Design review of the part built by this model. Coordinates are the model's own, in mm. Face numbers are marked on the shaded views. Give positions to 0.01 mm unless a question says otherwise; leave off trailing zeros. Loops run counter-clockwise (first coordinate to the right, second up) from the corner with the lowest first, then second, coordinate; pieces in that order, holes last. Notation, with made-up numbers: (-31.75, 83.5) -> (10.25, 83.5) arc R34 ccw to (10.25, 121.5) -> close; hole circle Ø10 at (50.25, -38.5). An arc over 180 degrees is marked (long way). Answer in a Markdown table with one row per item. Add a question column.
(1) Consider section B-B on y = 19.2. Write out the cut boundary in (x, z).
(2) Draft analysis for pull direction X (two halves, no side actions). For the marked faces 1, 2 and 3, state which applies: +X half, -X half, draft (parallel to the pull), parting line (faces both ways), or undercut.
(3) For pin 1 (8 mm diameter, centred on y = 9, z = -1, fed in from -X); pin 2 (1 mm diameter, centred on y = 8, z = 9.5, fed in from +X); pin 3 (6 mm diameter, centred on x = 4, y = 7.5, fed in from +Z); pin 4 (2.5 mm diameter, centred on x = 0, y = 19.2, fed in from -Z), all flat-tipped, find the tip position at first contact; note any pin that passes through.
(4) For line 1 (Y direction, x = 0, z = 8.5); line 2 (Z direction, x = 0, y = 2); line 3 (Z direction, x = 3.75, y = 5), list the stretches that pass through material, from the lowest coordinate up.
(5) Consider section C-C on y = 22.75. Write out the cut boundary in (x, z), then the cut area to 3 significant figures.
(6) Consider section D-D on x = 6.5. Write out the cut boundary in (y, z), then the cut area to 3 significant figures.
(7) Consider section A-A on z = 0. Write out the cut boundary in (x, y), then the cut area to 3 significant figures.
Autodesk Inventor part; units mm, degrees
ref_plane "YZ Plane" through (0, 0, 0) normal (1, 0, 0) x (0, 1, 0)
ref_plane "XZ Plane" through (0, 0, 0) normal (0, 1, 0) x (-1, 0, 0)
ref_plane "XY Plane" through (0, 0, 0) normal (0, 0, 1) x (1, 0, 0)
sketch "Boceto1" plane through (0, 0, 0) normal (0, 1, 0) x (-1, 0, 0)
  circle A0 centre (0, 0) radius 12
  dimension "d0" = 24
extrude "Extrusión1" add sketch "Boceto1" along normal blind 25.6
sketch "Boceto2" plane through (0, 25.6, 0) normal (0, 1, 0) x (1, 0, 0)
  point P0 (0, 0)
  point P1 (0, 0)
hole "Agujero1" at (0, 25.6, 0) direction (0, -1, 0) diameter 5 depth 35 tip angle 118
sketch "Boceto3" plane through (0, 25.6, 0) normal (0, 1, 0) x (1, 0, 0)
  point P0 (0, 0)
  point P1 (0, 0)
hole "Agujero2" at (0, 25.6, 0) direction (0, -1, 0) diameter 8 depth 12.8
sketch "Boceto4" plane through (0, 0, 0) normal (1, 0, 0) x (0, 1, 0)
  line L0 (9.2, -7) -> (3.6, -7)
  line L1 (3.6, -7) -> (3.6, -9.42)
  line L2 (3.6, -9.42) -> (9.2, -9.42)
  line L3 (9.2, -9.42) -> (9.2, -7)
  line L4 (25.6, -12) -> (25.6, 12) construction
  line L5 (0, 12) -> (0, -12) construction
  line L6 (12.8, -2.5) -> (12.8, 2.5) construction
  line L7 (0, -2.5) -> (0, 2.5) construction
  line L8 (19.2, 26.4321) -> (19.2, -18.0419) construction
  line L9 (6.4, 12.9466) -> (6.4, -18.0419) construction
  line L10 (22, -7) -> (16.4, -7)
  line L11 (16.4, -7) -> (16.4, -9.42)
  line L12 (16.4, -9.42) -> (22, -9.42)
  line L13 (22, -9.42) -> (22, -7)
  line L14 (0, -2.5) -> (0, 2.5) construction
  point P0 (0, 0)
  point P1 (6.4, -7)
  point P2 (19.2, -7)
  dimension "d17" = 5.6
  dimension "d18" = 2.42
  dimension "d19" = 6.4
  dimension "d20" = 6.4
  dimension "d21" = 5.6
  dimension "d22" = 2.42
  dimension "d23" = 9.42
  dimension "d24" = 9.42
extrude "Extrusión2" cut sketch "Boceto4" along normal blind 10 and the other way blind 3
sketch "Boceto5" plane through (9.7468, 16.4, -7) normal (0, 0, -1) x (-1, 0, 0)
  line L0 (0, -7.2) -> (2.3128, -7.2) construction
  line L1 (2.3128, -7.2) -> (2.3128, -12.8) construction
  line L2 (2.3128, -12.8) -> (0, -12.8) construction
  line L3 (0, -12.8) -> (0, -7.2) construction
  line L4 (0, 5.6) -> (2.3128, 5.6) construction
  line L5 (2.3128, 5.6) -> (2.3128, 0) construction
  line L6 (2.3128, 0) -> (0, 0) construction
  line L7 (0, 0) -> (0, 5.6) construction
  line L8 (21.7468, 9.2) -> (-2.2532, 9.2) construction
  line L9 (-2.2532, -16.4) -> (21.7468, -16.4) construction
  point P0 (9.7468, -16.4)
  point P1 (9.7468, 2.8)
  point P2 (9.7468, -10)
  point P3 (2.3128, -10)
  point P4 (2.3128, 2.8)
hole "Agujero3" at (0, 19.2, -7) at (0, 6.4, -7) direction (0, 0, 1) diameter 3 end through all both
sketch "Boceto6" plane through (0, 12.8, 0) normal (0, 1, 0) x (1, 0, 0)
  circle A0 centre (0, 0) radius 4 construction
  circle A1 centre (0, 0) radius 12 construction
  circle A2 centre (0, 0) radius 2.5 construction
  line L0 (1.5, -1.5) -> (-1.5, -1.5)
  line L1 (-1.5, -1.5) -> (-1.5, 1.5)
  line L2 (-1.5, 1.5) -> (1.5, 1.5)
  line L3 (1.5, 1.5) -> (1.5, -1.5)
  line L4 (-1.5, 1.5) -> (1.5, -1.5) construction
  line L5 (1.5, 1.5) -> (-1.5, -1.5) construction
  circle A3 centre (0, 0) radius 4
  dimension "d36" = 3
  dimension "d37" = 3
  dimension "d38" = 8
extrude "Extrusión3" add sketch "Boceto6" along normal up to surface (12.8 mm away)
equation "\"d20\" = d19"
properties part number "Coupler 5x8"
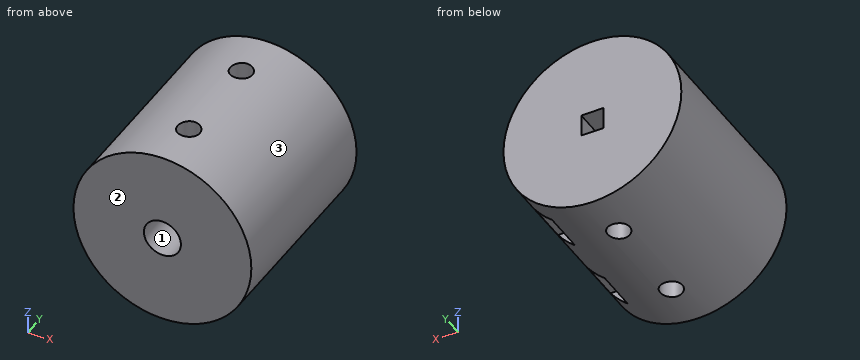
Values follow:
| question | item | result |
|---|---|---|
| 1 | outline | (-3, -9.42) -> (-3, -7) -> (-1.5, -7) -> (-1.5, -3.71) arc R4 ccw to (1.5, -3.71) -> (1.5, -7) -> (9.75, -7) arc R12 ccw to (1.5, 11.91) -> (1.5, 3.71) arc R4 ccw to (-1.5, 3.71) -> (-1.5, 11.91) arc R12 ccw to (-1.5, -11.91) -> (-1.5, -9.42) -> close; (1.5, -11.91) arc R12 ccw to (7.43, -9.42) -> (1.5, -9.42) -> close; hole (-1.5, -1.5) -> (1.5, -1.5) -> (1.5, 1.5) -> (-1.5, 1.5) -> close |
| 2 | face 1 | undercut |
| 2 | face 2 | draft |
| 2 | face 3 | parting line |
| 3 | pin 1 | x = -12 |
| 3 | pin 2 | x = 7.94 |
| 3 | pin 3 | z = 11.96 |
| 3 | pin 4 | z = -4 |
| 4 | line 1 | 0 to 4.9, 7.9 to 17.7, 20.7 to 25.6 |
| 4 | line 2 | -12 to -2.5, 2.5 to 12 |
| 4 | line 3 | -11.4 to -9.42, -7 to 11.4 |
| 5 | outline | circle Ø24 at (0, 0); hole (-1.5, -1.5) -> (1.5, -1.5) -> (1.5, 1.5) -> (-1.5, 1.5) -> close |
| 5 | area | 443 mm2 |
| 6 | outline | (0, -10.09) -> (25.6, -10.09) -> (25.6, 10.09) -> (0, 10.09) -> close; hole (3.6, -9.42) -> (9.2, -9.42) -> (9.2, -7) -> (3.6, -7) -> close; hole (16.4, -9.42) -> (22, -9.42) -> (22, -7) -> (16.4, -7) -> close |
| 6 | area | 489 mm2 |
| 7 | outline | (-12, 0) -> (-2.5, 0) -> (-2.5, 12.8) -> (-1.5, 12.8) -> (-1.5, 25.6) -> (-12, 25.6) -> close; (1.5, 12.8) -> (2.5, 12.8) -> (2.5, 0) -> (12, 0) -> (12, 25.6) -> (1.5, 25.6) -> close |
| 7 | area | 512 mm2 |
